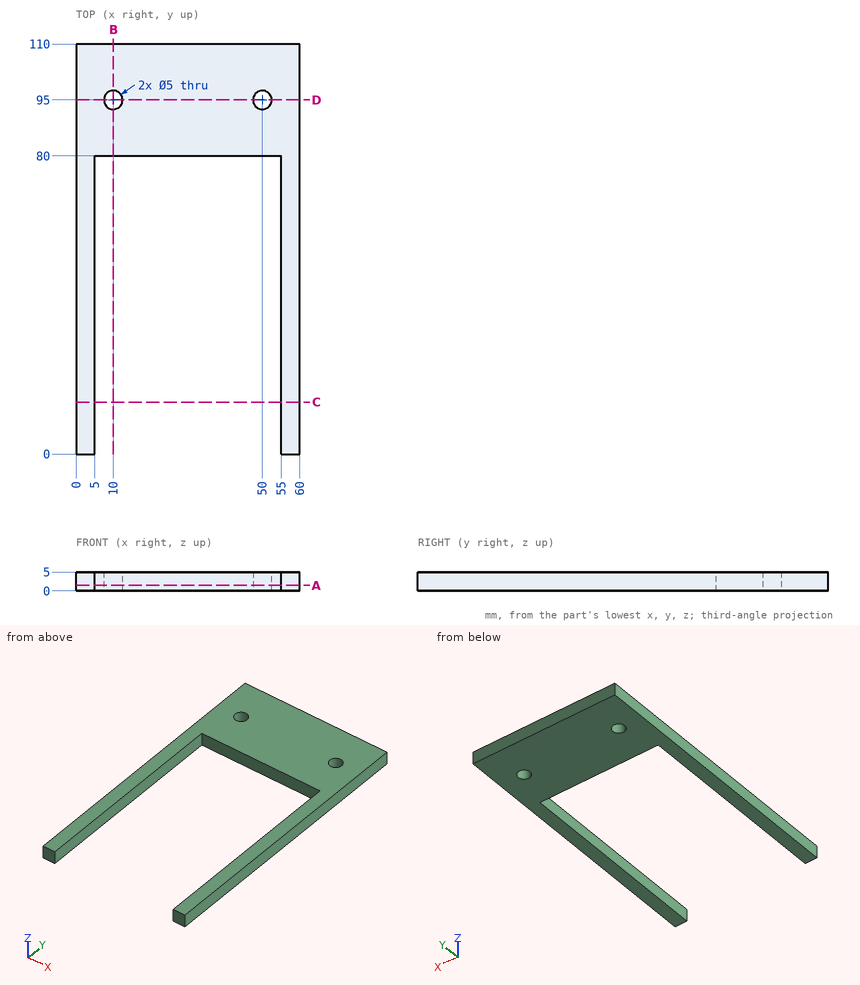
Job drawing, mm, ordinate dimensions from the low corner. One solid piece. Give positions to 0.01 mm unless a question says otherwise; leave off trailing zeros. Write each loop counter-clockwise with the first axis right and the second up, starting at its lowest first coordinate (ties: lowest second). Pieces come first, ordered by that corner, then holes. Notation, with made-up numbers: M -2,4.5 L 2,4.5 A28 ccw 2,34.5 Z; hole C 75.25,54 d2. An arc over 180 degrees is marked long. One line per item, written item: value. Start each with the question number.
Q1. Saw through at C-C, the plane y = 14. Write the cut outline in (x, z), plus the area to 3 significant figures.
Q2. Probe probe 1 along Y at (x, z) = (50, 3.4); probe 2 along X at (y, z) = (58.5, 4.7); probe 3 along Y at (x, z) = (54.5, 2.85). List the from-to ranges inside material, lowest first. Write a range as [from, to].
Q3. Saw through at A-A, the plane z = 1.5. Write the cut outline in (x, y).
Q4. Saw through at D-D, the plane y = 95. Write the cut outline in (x, z), plus the area to 3 significant figures.
Q5. Saw through at B-B, the plane x = 10. Write the cut outline in (y, z), plus the area to 3 significant figures.
Output values:
1. outline: M 0,0 L 5,0 L 5,5 L 0,5 Z; M 55,0 L 60,0 L 60,5 L 55,5 Z
1. area: 50.0 mm²
2. probe 1: y = [80, 92.5], [97.5, 110]
2. probe 2: x = [0, 5], [55, 60]
2. probe 3: y = [80, 110]
3. outline: M 0,0 L 5,0 L 5,80 L 55,80 L 55,0 L 60,0 L 60,110 L 0,110 Z; hole C 10,95 d5; hole C 50,95 d5
4. outline: M 0,0 L 7.5,0 L 7.5,5 L 0,5 Z; M 12.5,0 L 47.5,0 L 47.5,5 L 12.5,5 Z; M 52.5,0 L 60,0 L 60,5 L 52.5,5 Z
4. area: 250 mm²
5. outline: M 80,0 L 92.5,0 L 92.5,5 L 80,5 Z; M 97.5,0 L 110,0 L 110,5 L 97.5,5 Z
5. area: 125 mm²
